```python
from build123d import *

# Parameters (mm, degrees)
FDM_4MM_START                 = -32
FDM_4MM_DEPTH                 = 64
EXTRUDE_START                 = -30
EXTRUDE_45_1_DEPTH            = 12
CUT_EXTRUDE_M3_1_DEPTH        = 100
CUT_EXTRUDE_M3_1_DEPTH_BACK   = 100
SKETCH_3_R                    = 1.65
EXTRUDE_START_2               = 18
EXTRUDE_45_1_2_DEPTH          = 12
CUT_EXTRUDE_M3_1_2_DEPTH      = 100
CUT_EXTRUDE_M3_1_2_DEPTH_BACK = 100
SKETCH_5_R                    = 1.65
CUT_EXTRUDE_M3_1_3_DEPTH      = 100
CUT_EXTRUDE_M3_1_3_DEPTH_BACK = 100
SKETCH_6_R                    = 1.65
CUT_EXTRUDE_M3_1_4_DEPTH      = 100
CUT_EXTRUDE_M3_1_4_DEPTH_BACK = 100
SKETCH_7_R                    = 1.65


with BuildPart() as part:
    # 草图1 → FDM侧板连接根部_4mm壁 (new body)
    with BuildSketch(Plane.XY.offset(FDM_4MM_START)):
        Polygon((0, 0), (12, 0), (12, 4), (4, 4), (4, 14), (0, 14), align=None)
    extrude(amount=FDM_4MM_DEPTH)

    # 草图2 → Extrude 45__-1 (add)
    with BuildSketch(Plane.XY.offset(EXTRUDE_START)):
        Polygon((0, 0), (0, 14), (4, 14), (4, 0), (13, 0), (14.5, -1.5), (38.5, -25.5), (35.671572875, -28.328427125), (11.671572875, -4.328427125), (0, -4.328427125), align=None)
    extrude(amount=EXTRUDE_45_1_DEPTH)

    # 草图3 → Cut-Extrude M3__-1 (cut, two sides: drawn at the far end of the back side and taken through both)
    with BuildSketch(Plane(origin=(0, 0, 0), x_dir=(0, 0, -1), z_dir=(1, 0, 0)).offset(-CUT_EXTRUDE_M3_1_DEPTH_BACK)):
        with Locations((24, 10)):
            Circle(SKETCH_3_R)
    extrude(amount=CUT_EXTRUDE_M3_1_DEPTH + CUT_EXTRUDE_M3_1_DEPTH_BACK, mode=Mode.SUBTRACT)

    # 草图4 → Extrude 45__1 2 (add)
    with BuildSketch(Plane.XY.offset(EXTRUDE_START_2)):
        Polygon((0, 0), (0, 14), (4, 14), (4, 0), (13, 0), (14.5, -1.5), (38.5, -25.5), (35.671572875, -28.328427125), (11.671572875, -4.328427125), (0, -4.328427125), align=None)
    extrude(amount=EXTRUDE_45_1_2_DEPTH)

    # 草图5 → Cut-Extrude M3__1 2 (cut, two sides: drawn at the far end of the back side and taken through both)
    with BuildSketch(Plane(origin=(0, 0, 0), x_dir=(0, 0, -1), z_dir=(1, 0, 0)).offset(-CUT_EXTRUDE_M3_1_2_DEPTH_BACK)):
        with Locations((-24, 10)):
            Circle(SKETCH_5_R)
    extrude(amount=CUT_EXTRUDE_M3_1_2_DEPTH + CUT_EXTRUDE_M3_1_2_DEPTH_BACK, mode=Mode.SUBTRACT)

    # 草图6 → Cut-Extrude M3_-1 3 (cut, two sides: drawn at the far end of the back side and taken through both)
    with BuildSketch(Plane(origin=(6.5, 6.5, 0), x_dir=(0, 0, -1), z_dir=(0.7071067811865472, 0.7071067811865479, 0)).offset(-CUT_EXTRUDE_M3_1_3_DEPTH_BACK)):
        with Locations(Location((24, -35.813708499, 0), (0, 0, 90))):
            Circle(SKETCH_6_R)
    extrude(amount=CUT_EXTRUDE_M3_1_3_DEPTH + CUT_EXTRUDE_M3_1_3_DEPTH_BACK, mode=Mode.SUBTRACT)

    # 草图7 → Cut-Extrude M3_1 4 (cut, two sides: drawn at the far end of the back side and taken through both)
    with BuildSketch(Plane(origin=(6.5, 6.5, 0), x_dir=(0, 0, -1), z_dir=(0.7071067811865472, 0.7071067811865479, 0)).offset(-CUT_EXTRUDE_M3_1_4_DEPTH_BACK)):
        with Locations(Location((-24, -35.813708499, 0), (0, 0, 90))):
            Circle(SKETCH_7_R)
    extrude(amount=CUT_EXTRUDE_M3_1_4_DEPTH + CUT_EXTRUDE_M3_1_4_DEPTH_BACK, mode=Mode.SUBTRACT)


solid = part.part
```
Input: part model. Units: mm. Frame: model coordinates. A direction names the side the tool comes from. Give positions to 0.01 mm unless a question says otherwise; leave off trailing zeros. Order: outer loops, then holes, each group sorted by start corner. A loop starts at its lowest first (then second) coordinate and runs counter-clockwise, first axis right, second up.
1. Pin query (flat end, axial travel): pin 1 Ø0.8 at (x, z) = (12.5, -21.5) entering from +Y; pin 2 Ø2 at (x, z) = (11, -7) entering from +Y; pin 3 Ø4.5 at (y, z) = (10, -24) entering from +X. Return the tip coordinate at first contact, or that it passes through.
Computed:
pin 1: stops at y = 0
pin 2: stops at y = 4
pin 3: stops at x = 4
2. Cut plane D-D (z = 24). Return loops of the section in (x, y), and give its area (3 significant figures).
Computed:
outline: (0, -4.33) - (11.67, -4.33) - (27.83, -20.49) - (30.66, -17.66) - (13, 0) - (12, 0) - (12, 4) - (4, 4) - (4, 8.35) - (0, 8.35) - close; (0, 11.65) - (4, 11.65) - (4, 14) - (0, 14) - close; (30.16, -22.82) - (35.67, -28.33) - (38.5, -25.5) - (32.99, -19.99) - close
area: 255 mm2
3. Draft query along Z for faces 4 (the face through (21, -11, 30)), 5 (the face through (29.76, -19.63, 25.39)), 6 (the face through (26, -13, 24)). Return one class per face: released by +Z, released by -Z, zero draft, split by the parting line, or undercut.
Computed:
face 4: released by +Z
face 5: undercut
face 6: zero draft
4. Cut plane C-C (x = 22.5). Return loops of the section in (y, z).
Computed:
outline: (-15.16, -30) - (-9.5, -30) - (-9.5, -18) - (-15.16, -18) - close; (-15.16, 18) - (-9.5, 18) - (-9.5, 30) - (-15.16, 30) - close
5. Cut plane B-B (y = -3.5). Return loops of the section in (x, z), and give its area (3 significant figures).
Computed:
outline: (0, -30) - (16.5, -30) - (16.5, -18) - (0, -18) - close; (0, 18) - (16.5, 18) - (16.5, 30) - (0, 30) - close
area: 396 mm2
6. Line query: probe 1 along Z at (x, y) = (2.55, 10); probe 2 along Y at (x, z) = (2, -24); probe 3 along Z at (x, y) = (15, -4). Output: solid intervals per line, ascending.
Computed:
probe 1: z = -32 to -25.65, -22.35 to 22.35, 25.65 to 32
probe 2: y = -4.33 to 8.35, 11.65 to 14
probe 3: z = -30 to -18, 18 to 30
7. Set-up query: faces 1 (the face through (8, 4, 0)), 2 (the face through (6, -4.328, -24)), 3 (the face through (6, 0, 0)). Return all of +Z, -Z, +X, -X, +Y, -Y with unobstructed straight access to the full face (end or side cutting, diameter ignored); none if empty.
Computed:
face 1: +Z, -Z, +X, +Y
face 2: +Z, -Z, -X, -Y
face 3: +X, -X, -Y
8. Cut plane A-A (y = 10). Return loops of the section in (x, z).
Computed:
outline: (0, -32) - (4, -32) - (4, -25.65) - (0, -25.65) - close; (0, -22.35) - (4, -22.35) - (4, 22.35) - (0, 22.35) - close; (0, 25.65) - (4, 25.65) - (4, 32) - (0, 32) - close
